The model under review builds one solid part; all positions refer to its coordinate system, in mm. Face numbers are marked on the shaded views. Give positions to 0.01 mm unless a question says otherwise; leave off trailing zeros. Order: outer loops, then holes, each group sorted by start corner. A loop starts at its lowest first (then second) coordinate and runs counter-clockwise, first axis right, second up. Notation, with made-up numbers: (-28.75, 56.25) - (9.25, 56.25) arc R13 cw to (9.25, 71.25) - close; hole circle Ø5 at (-18, 59.5). An arc over 180 degrees is marked (long way). Put each result on its own line as item: value.
```python
from build123d import *

# Parameters (mm, degrees)
F2_R     = 5.08
F4_DEPTH = 1.905
F6_DEPTH = 5.08
F7_R     = 1.905
F7_W     = 7.62
F7_H     = 2.54
F8_DEPTH = 10.16


with BuildPart() as f1:
    # F0 (on Front) → F1 (revolve)
    with BuildSketch(Plane.XZ):
        Polygon((12.7, 50.8), (12.7, 0), (25.4, 0), (19.05, 31.75), (25.4, 50.8), align=None)
    revolve(axis=Axis((12.7, 0, 25.4), (0, 0, -1)))

    # F2
    f2_edges = [f1.edges().sort_by_distance(p)[0] for p in [
        (0, 0, 50.8),
        (6.35, 0, 31.75),
    ]]
    fillet(f2_edges, radius=F2_R)

    # F3 (on Front) → F4 (join, symmetric)
    with BuildSketch(Plane.XZ):
        Polygon((2.54, 60.96), (7.62, 50.8), (17.78, 50.8), (22.86, 60.96), (12.7, 71.12), align=None)
    extrude(amount=F4_DEPTH, both=True)

    # F5 (on Front) → F6 (join, symmetric)
    with BuildSketch(Plane.XZ):
        Polygon((11.43, 63.5), (8.89, 63.5), (8.89, 60.96), (11.43, 60.96), (11.43, 50.8), (13.97, 50.8), (13.97, 60.96), (16.51, 60.96), (16.51, 63.5), (13.97, 63.5), (13.97, 66.04), (11.43, 66.04), align=None)
    extrude(amount=F6_DEPTH, both=True)

    # F7 (on Front) → F8 (join)
    with BuildSketch(Plane.XZ):
        with Locations((7.62, 40.3035629486)):
            Circle(F7_R)
        with Locations((17.78, 40.3035629486)):
            Circle(F7_R)
        with Locations((12.7, 36.4935629486)):
            Rectangle(F7_W, F7_H)
    extrude(amount=F8_DEPTH)


solid = f1.part
```
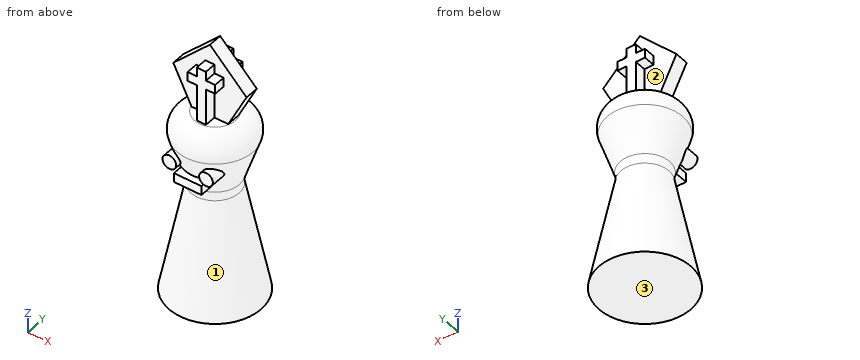
(1) Take a section at A-A, the plane z = 26. Write out the cut boundary in (x, y), then the cut area to 3 significant figures.
The answers:
outline: circle Ø15 at (12.7, 0)
area: 177 mm^2
(2) Wall thickness on L1, parallel to Z at x = 8, y = -3.75; L2, parallel to Z at x = 15.75, y = -5; L3, parallel to Y at x = 7.25, z = 59.5 (3 decimals): over which ranges is each line inside the solid? List them lowest first.
The answers:
L1: 0 to 50.79
L2: 0 to 50.8, 60.96 to 63.5
L3: -1.905 to 1.905
(3) The part is to be moulded in two halves that separate along Z. For the marked faces 1, 2 and 3, say which applies: pulls with the +Z half, pulls with the -Z half, needs draft (parallel to the pull), parting line crosses it, or undercut.
The answers:
face 1: undercut
face 2: undercut
face 3: pulls with the -Z half
(4) Take a section at B-B, the plane z = 13. Write out the cut boundary in (x, y).
The answers:
outline: circle Ø20.2 at (12.7, 0)
(5) Clearance check with flat-ended pins moving along their axes: pin 1 Ø1.5 at (x, y) = (4.5, 10) entering from -Z; pin 2 Ø10 at (y, z) = (2.5, 28.5) entering from -X; pin 3 Ø1.3 at (y, z) = (4, 65) entering from -X; pin 4 Ø0.8 at (y, z) = (3.5, 62.5) entering from -X. State where each tip first meets the part, or that it passes through.
The answers:
pin 1: z = 0
pin 2: x = 4.8
pin 3: x = 11.43
pin 4: x = 8.89
